from build123d import *

# Parameters (mm, degrees)
F0_W     = 46.9405390322
F0_H     = 38.6983044446
F1_DEPTH = 38.1
F3_W     = 19.05
F3_H     = 19.7009555995
F4_DEPTH = 25.4
F5_DEPTH = 50.8


with BuildPart() as f1:
    # F0 (on Front) → F1 (new body)
    with BuildSketch(Plane.XZ):
        with Locations((23.4702695161, 19.3491522223)):
            Rectangle(F0_W, F0_H)
    extrude(amount=F1_DEPTH)

    # F3 (on face) → F4 (cut)
    with BuildSketch(Plane(origin=(0, 0, 0), x_dir=(0, -1, 0), z_dir=(-1, 0, 0))):
        with Locations((28.575, 28.8478266448)):
            Rectangle(F3_W, F3_H)
    extrude(amount=-F4_DEPTH, mode=Mode.SUBTRACT)

    # F5 (cut): a face of the model
    f5_faces = [f1.faces().sort_by_distance(p)[0] for p in [
        (25.4, -28.575, 28.8478266448),
    ]]
    extrude(f5_faces, amount=-F5_DEPTH, mode=Mode.SUBTRACT)


solid = f1.part
For this review, take the finished solid that the model builds, in its own axes (mm). A direction names the side the tool comes from. Give positions to 0.01 mm unless a question says otherwise; leave off trailing zeros. Loops run counter-clockwise (first coordinate to the right, second up) from the corner with the lowest first, then second, coordinate; pieces in that order, holes last. Notation, with made-up numbers: (80, 8.5) - (104, 8.5) arc R13 ccw to (104, 23.5) - close; hole circle Ø1 at (28.25, -24.75). An arc over 180 degrees is marked (long way). Write each question's results on one line, items separated by ' | '.
(1) For line 1 along Z through (x, y) = (24.5, -28); line 2 along Y through (x, z) = (20.5, 35.5), list the stretches that pass through material, from the lowest coordinate up.
Conclusion:
line 1: 0 to 19 | line 2: -19.05 to 0
(2) Take a section at B-B (z = 25). Give the boundary of the cut face in (x, y), then the cut area to 3 significant figures.
Conclusion:
outline: (0, -19.05) - (46.94, -19.05) - (46.94, 0) - (0, 0) - close | area: 894 mm^2
(3) For pin 1 Ø10 at (x, y) = (16.5, -29) entering from +Z; pin 2 Ø21.5 at (x, z) = (30.5, 32.5) entering from -Y, all flat-tipped, find the tip position at first contact; note any pin that passes through.
Conclusion:
pin 1: z = 19 | pin 2: y = -19.05
(4) Take a section at C-C (y = -21.5). Give the boundary of the cut face in (x, z), then the cut area to 3 significant figures.
Conclusion:
outline: (0, 0) - (46.94, 0) - (46.94, 19) - (0, 19) - close | area: 892 mm^2
(5) Take a section at A-A (x = 23). Give the boundary of the cut face in (y, z).
Conclusion:
outline: (-38.1, 0) - (0, 0) - (0, 38.7) - (-19.05, 38.7) - (-19.05, 19) - (-38.1, 19) - close
(6) For faces 1 (the flat face through (0, -15, 15)), 2 (the flat face through (23, -19.05, 29)), list the 3-axis set-ups (+Z, -Z, +X, -X, +Y, -Y) from which the entire face can be reached by the end or side of a thin tool; tool diameter is ignored.
Conclusion:
face 1: +Z, -Z, -X, +Y, -Y | face 2: +Z, +X, -X, -Y
